Read the model definition and answer for the solid it produces. Units are mm, in the model's axes. Round coordinates to 2 decimals unless told otherwise and drop trailing zeros. Loops run counter-clockwise (first coordinate to the right, second up) from the corner with the lowest first, then second, coordinate; pieces in that order, holes last. Notation, with made-up numbers: (-19.75, -40) - (-3.75, -40) arc R24 cw to (-3.75, -23) - close; hole circle Ø7 at (46, -5.5). An arc over 180 degrees is marked (long way). Use CSV: the item, a comma, the result in double quotes. Start each with the question number.
1. Find section C-C (x = 13). Give the vertices of the cut face in (y, z), and give its area (3 significant figures).
2. Given pin 1 Ø6 at (x, z) = (15.5, 9) entering from +Y; pin 2 Ø6 at (x, z) = (28, 15.5) entering from +Y, each flat-ended and moving along its own axis, determine where each tip first touches the part or whether it passes through.
3. Find section A-A (z = 20). Give the vertices of the cut face in (x, y), and give its area (3 significant figures).
4. Find section B-B (y = 11.25). Give the vertices of the cut face in (x, z).
5. Consider line 1 along Y through (x, z) = (25.5, 20.25); line 2 along Y through (x, z) = (7, 10.25); line 3 along X through (y, z) = (10.5, 22.75). Determine where each line is inside the solid, lowest interval first.
Autodesk Inventor part; units mm, degrees
ref_plane "YZ Plane" through (0, 0, 0) normal (1, 0, 0) x (0, 1, 0)
ref_plane "XZ Plane" through (0, 0, 0) normal (0, 1, 0) x (-1, 0, 0)
ref_plane "XY Plane" through (0, 0, 0) normal (0, 0, 1) x (1, 0, 0)
sketch "Sketch1" plane through (0, 0, 0) normal (0, 0, 1) x (1, 0, 0)
  line L0 (0, 0) -> (32.4623, 0)
  line L1 (32.4623, 0) -> (32.4623, 18.6079)
  line L2 (32.4623, 18.6079) -> (0, 18.6079)
  line L3 (0, 18.6079) -> (0, 0)
extrude "Extrusion1" add sketch "Sketch1" along normal blind 25.4
sketch "Sketch2" plane through (0, 0, 25.4) normal (0, 0, 1) x (1, 0, 0)
  line L0 (32.4623, 0) -> (32.4623, 18.6079)
  line L1 (32.4623, 18.6079) -> (0, 18.6079)
  line L2 (6.7125, 18.6079) -> (32.4623, 6.0135)
extrude "Extrusion2" cut sketch "Sketch2" against normal through all
properties part number "Work Planes"
Filled sheet:
1,outline,"(0, 0) - (15.53, 0) - (15.53, 25.4) - (0, 25.4) - close"
1,area,"395 mm²"
2,pin 1,"stops at y = 15.78"
2,pin 2,"stops at y = 9.66"
3,outline,"(0, 0) - (32.46, 0) - (32.46, 6.01) - (6.71, 18.61) - (0, 18.61) - close"
3,area,"442 mm²"
4,outline,"(0, 0) - (21.76, 0) - (21.76, 25.4) - (0, 25.4) - close"
5,line 1,"y = 0 to 9.42"
5,line 2,"y = 0 to 18.47"
5,line 3,"x = 0 to 23.29"
